Design review of the part built by this model. Coordinates are the model's own, in mm. Face numbers are marked on the shaded views. A direction names the side the tool comes from. Coordinates: 2 decimals unless noted, no trailing zeros. Write each loop counter-clockwise with the first axis right and the second up, starting at its lowest first coordinate (ties: lowest second). Pieces come first, ordered by that corner, then holes. Notation, with made-up numbers: M 68.5,-16 L 90.5,-16 A31 cw 90.5,11 Z; hole C -37,9 d9. An arc over 180 degrees is marked long. Write item = value, one per line.
```python
from build123d import *

# Parameters (mm, degrees)
F1_DEPTH = 25.4
F2_R     = 5.08
F3_R     = 1.5875
F4_W     = 9
F4_H     = 28.575
F5_DEPTH = 127
F6_R     = 1.524
F7_R     = 15.875
F8_DEPTH = 152.4
F9_R     = 5.08


with BuildPart() as f1:
    # F0 (on Right) → F1 (new body, symmetric)
    with BuildSketch(Plane.YZ):
        Polygon((68.2625, -73.025), (68.2625, 73.025), (-30.1625, 73.025), (-30.1625, -9.525), (-68.2625, -12.7), (-68.2625, -73.025), align=None)
    extrude(amount=F1_DEPTH, both=True)

    # F2
    f2_edges = [f1.edges().sort_by_distance(p)[0] for p in [
        (0, -68.2625, -12.7),
        (0, -30.1625, -9.525),
        (0, -30.1625, 73.025),
        (0, 68.2625, 73.025),
        (0, 68.2625, -73.025),
        (0, -68.2625, -73.025),
    ]]
    fillet(f2_edges, radius=F2_R)

    # F3
    f3_edges = [f1.edges().sort_by_distance(p)[0] for p in [
        (25.4, -49.2125, -11.1125),
        (-25.4, -49.2125, -11.1125),
    ]]
    fillet(f3_edges, radius=F3_R)

    # F4 (on face) → F5 (join)
    with BuildSketch(Plane.XZ.offset(68.2625)):
        with Locations((0, -42.8625)):
            Rectangle(F4_W, F4_H)
    extrude(amount=F5_DEPTH)

    # F6
    f6_edges = [f1.edges().sort_by_distance(p)[0] for p in [
        (4.5, -131.7625, -28.575),
        (-4.5, -131.7625, -28.575),
        (4.5, -131.7625, -57.15),
        (-4.5, -131.7625, -57.15),
    ]]
    fillet(f6_edges, radius=F6_R)

    # F7 (on face) → F8 (join)
    with BuildSketch(Plane.XZ.offset(30.1625)):
        with Locations((0, 28.575)):
            Circle(F7_R)
    extrude(amount=F8_DEPTH)

    # F9
    f9_edges = [f1.edges().sort_by_distance(p)[0] for p in [
        (-15.875, -182.5625, 28.575),
    ]]
    fillet(f9_edges, radius=F9_R)


solid = f1.part
```
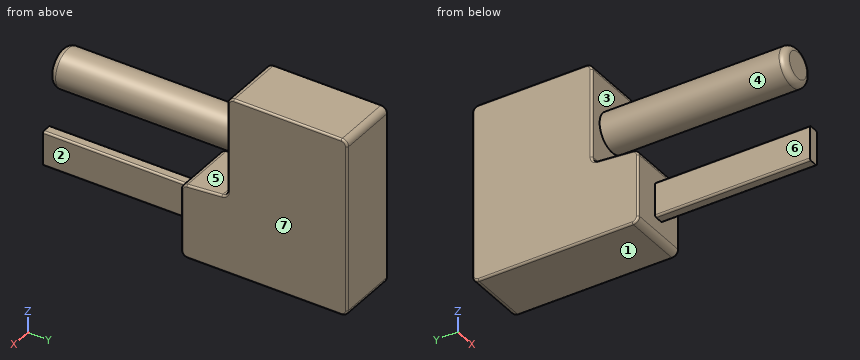
Q1. Machinability: for the marked faces 4, 5, 6 and 7, which of the approach directions +Z, -Z, +X, -X, +Y, -Y give a long, thin tool a straight path to every point of the face, cutting with its end or side? Answer none if there is none.
Check result:
face_4 = -Y
face_5 = +X, -X, -Y
face_6 = -Z, -X, -Y
face_7 = +Z, -Z, +X, +Y, -Y
Q2. Consider section C-C, the plane z = 58.5. State the section outline as (x, y) points (1 decimal), and give its area (3 significant figures).
Check result:
outline = M -25.4,-28.6 A1.6 ccw -23.8,-30.2 L 23.8,-30.2 A1.6 ccw 25.4,-28.6 L 25.4,66.7 A1.6 ccw 23.8,68.3 L -23.8,68.3 A1.6 ccw -25.4,66.7 Z
area = 5,000 mm²
Q3. Consider section B-B, the plane z = -24. State the section outline as (x, y) points (1 decimal), and give its area (3 significant figures).
Check result:
outline = M -25.4,-66.7 A1.6 ccw -23.8,-68.3 L 23.8,-68.3 A1.6 ccw 25.4,-66.7 L 25.4,66.7 A1.6 ccw 23.8,68.3 L -23.8,68.3 A1.6 ccw -25.4,66.7 Z
area = 6,930 mm²
Q4. Consider section D-D, the plane z = -46. State the section outline as (x, y) points (1 decimal).
Check result:
outline = M -25.4,-66.7 A1.6 ccw -23.8,-68.3 L -4.5,-68.3 L -4.5,-195.3 L 4.5,-195.3 L 4.5,-68.3 L 23.8,-68.3 A1.6 ccw 25.4,-66.7 L 25.4,66.7 A1.6 ccw 23.8,68.3 L -23.8,68.3 A1.6 ccw -25.4,66.7 Z
Q5. Wall thickness on line 1 (Z direction, x = 0, y = -127.5) (3 decimals); line 2 (Y direction, x = -4, z = -4.5); line 3 (Y direction, x = 6.5, z = -63.5): over which ranges is each line inside the solid? List them lowest first.
Check result:
line_1 = -57.15 to -28.575, 12.7 to 44.45
line_2 = -30.16 to 68.26
line_3 = -68.26 to 68.26
Q6. The part is to be moulded in two halves that separate along Z. For the marked faces 1, 2 and 3, say which applies: +Z half, -Z half, draft (parallel to the pull), parting line (faces both ways), or undercut.
Check result:
face_1 = -Z half
face_2 = draft
face_3 = undercut
Q7. For P1, Ø1, axis at x = -5.5, y = -168, coming from the +Z side; P2, Ø5, axis at x = -6, y = -142, coming from the -Z side; P3, Ø5, axis at x = 19, z = -4.5, coming from the -Y side, all flat-tipped, find the tip position at first contact; note any pin that passes through.
Check result:
P1 = 43.64
P2 = -57.06
P3 = -30.64
